Build history of the part. All positions in model axes, mm. Give positions to 0.01 mm unless a question says otherwise; leave off trailing zeros. Loops run counter-clockwise (first coordinate to the right, second up) from the corner with the lowest first, then second, coordinate; pieces in that order, holes last. Notation, with made-up numbers: (-33.5, 49.5) -> (-15.5, 49.5) arc R25 ccw to (-15.5, 71.5) -> close; hole circle Ø9 at (39.5, 22). An arc over 180 degrees is marked (long way). Answer as a JSON object with one key per item and string values. Group by question number.
from build123d import *

# Parameters (mm, degrees)
F0_W     = 80
F0_H     = 60
F1_DEPTH = 50.8
F2_W     = 5
F2_H     = 30
F3_DEPTH = 40
F4_R     = 0.5
F5_R     = 0.505
F6_DEPTH = 45


with BuildPart() as f1:
    # F0 (on Top) → F1 (new body)
    with BuildSketch(Plane.XY):
        Rectangle(F0_W, F0_H)
    extrude(amount=F1_DEPTH)

    # F2 (on face) → F3 (cut)
    with BuildSketch(Plane.XY.offset(50.8)):
        with Locations((-20, 0)):
            Rectangle(F2_W, F2_H)
    extrude(amount=-F3_DEPTH, mode=Mode.SUBTRACT)

    # F4
    f4_edges = [f1.edges().sort_by_distance(p)[0] for p in [
        (-22.5, 15, 30.8),
        (-17.5, 15, 30.8),
        (-22.5, -15, 30.8),
        (-17.5, -15, 30.8),
    ]]
    fillet(f4_edges, radius=F4_R)

    # F5 (on face) → F6 (cut)
    with BuildSketch(Plane.XY.offset(50.8)):
        with Locations((20.357101, 0)):
            Circle(F5_R)
    extrude(amount=-F6_DEPTH, mode=Mode.SUBTRACT)


solid = f1.part
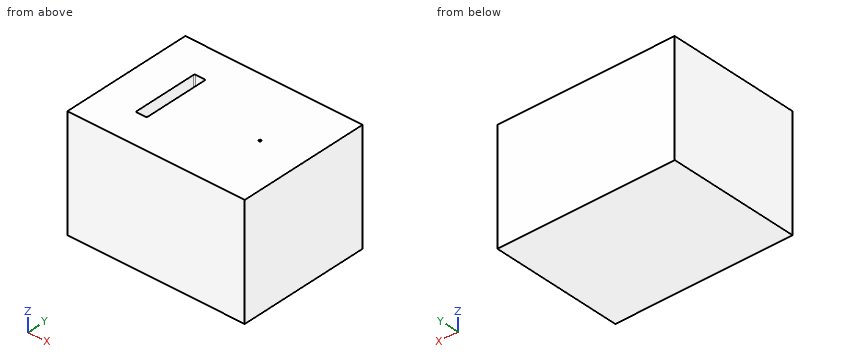
(1) Saw through at B-B on z = 43.5. List the corners of the cut face in (x, y) (3 decimals).
(2) Probe line 1 along Y through (x, z) = (-21, 39); line 2 along X through (y, z) = (4.5, 18.5). List the from-to ranges inside material, lowest first. Write a range as [from, to].
(3) Saw through at A-A on y = -13. List the corners of the cut face in (x, z), plus the area to 3 significant figures.
(4) Pin check, flat tips, straight feed: pin 1 (12 mm diameter, centred on x = -5.5, y = 1.5, fed in from -Z); pin 2 (0.9 mm diameter, centred on x = 20.36, y = 0, fed in from +Z); pin 3 (1.5 mm diameter, centred on x = -19, y = 3, fed in from +Z). Stop position of each tip, or through.
Calculated:
{
 "1": {"outline": "(-40, -30) -> (40, -30) -> (40, 30) -> (-40, 30) -> close; hole (-22.5, -14.5) arc R0.5 ccw to (-22, -15) -> (-18, -15) arc R0.5 ccw to (-17.5, -14.5) -> (-17.5, 14.5) arc R0.5 ccw to (-18, 15) -> (-22, 15) arc R0.5 ccw to (-22.5, 14.5) -> close; hole circle Ø1.01 at (20.357, 0)"},
 "2": {"line 1": "y = [-30, -15], [15, 30]", "line 2": "x = [-40, -22.5], [-17.5, 40]"},
 "3": {"outline": "(-40, 0) -> (40, 0) -> (40, 50.8) -> (-17.5, 50.8) -> (-17.5, 10.8) -> (-22.5, 10.8) -> (-22.5, 50.8) -> (-40, 50.8) -> close", "area": "3,860 mm^2"},
 "4": {"pin 1": "stops at z = 0", "pin 2": "stops at z = 5.8", "pin 3": "stops at z = 10.8"}
}
